Source: three-view drawing plus pictorial views. Frame: mm from the lowest corner of the part. A direction names the side the tool comes from. Give positions to 0.01 mm unless a question says otherwise; leave off trailing zeros. Order: outer loops, then holes, each group sorted by start corner. A loop starts at its lowest first (then second) coordinate and runs counter-clockwise, first axis right, second up. Notation, with made-up numbers: M 36,-18.5 L 83,-18.5 A19 cw 83,-10.5 Z; hole C 16,62.25 d2. An arc over 180 degrees is marked long. Use CSV: the item, a comma, the result in double quotes. Start each with the question number.
1. Section query B-B, the plane x = 24. Return the cut outline in (y, z), plus the area to 3 significant figures.
2. Mould query, pull axis Y, two halves, no side actions, for the marked faces 1, 2, 3 and 4. Classes: released by +Y, released by -Y, zero draft, split by the parting line, or undercut.
3. Section query A-A, the plane z = 12. Return the cut outline in (x, y), plus the area to 3 significant figures.
4. Section query C-C, the plane y = 24. Return the cut outline in (x, z), plus the area to 3 significant figures.
5. Reachability of the marked faces 5, 6 and 7 from +Z, -Z, +X, -X, +Y, -Y: full face, straight path, thin tool, end or side. Return the list, or none.
6. Line query: line 1 along Z through (x, y) = (24, 28.45); line 2 along Y through (x, z) = (23, 9.5); line 3 along Y through (x, z) = (36.5, 38). Output: solid intervals per line, ascending. Write a range as [from, to].
7. Section query D-D, the plane z = 4.5. Return the cut outline in (x, y).
8. Pin query (flat end, axial travel): P1, Ø6, axis at x = 26.5, z = 6.5, coming from the -Y side; P2, Ø1.5, axis at y = 20, z = 13.5, coming from the +X side; P3, Ø10, axis at x = 37, z = 13.5, coming from the -Y side; P4, Ø22, axis at x = 26, y = 23.5, coming from the -Z side. Return the tip coordinate at first contact, or that it passes through.
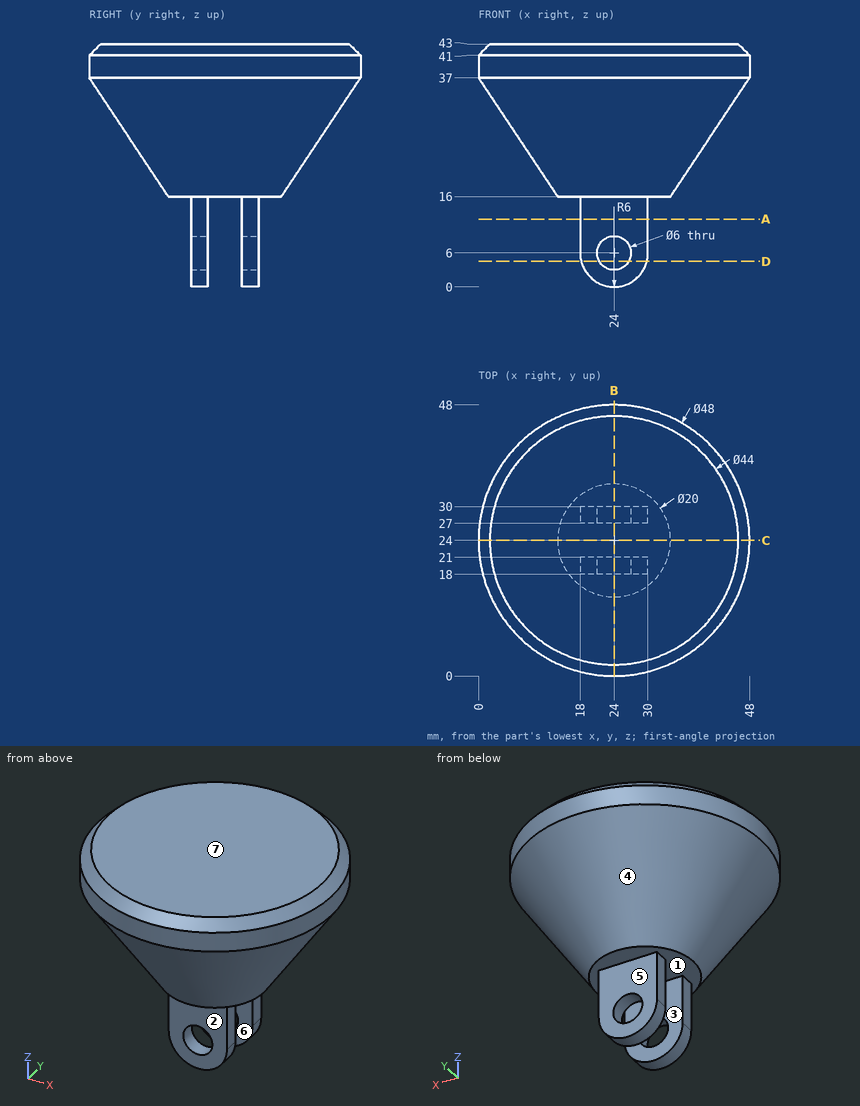
Result set:
1,outline,"M 0,37 L 14,16 L 18,16 L 18,9 L 21,9 L 21,16 L 27,16 L 27,9 L 30,9 L 30,16 L 34,16 L 48,37 L 48,41 L 46,43 L 2,43 L 0,41 Z; M 18,0 L 21,0 L 21,3 L 18,3 Z; M 27,0 L 30,0 L 30,3 L 27,3 Z"
1,area,"1,060 mm2"
2,face 1,"undercut"
2,face 2,"released by -Y"
2,face 3,"undercut"
2,face 4,"split by the parting line"
3,outline,"M 18,18 L 30,18 L 30,21 L 18,21 Z; M 18,27 L 30,27 L 30,30 L 18,30 Z"
3,area,"72.0 mm2"
4,outline,"M 0,37 L 14,16 L 34,16 L 48,37 L 48,41 L 46,43 L 2,43 L 0,41 Z"
4,area,"998 mm2"
5,face 5,"-Z, +X, -X, +Y"
5,face 6,"-Z, +X, -X"
5,face 7,"+Z, +X, -X, +Y, -Y"
6,line 1,"[0, 3], [9, 43]"
6,line 2,"[18, 21], [27, 30]"
6,line 3,"[3.51, 44.49]"
7,outline,"M 18.19,18 L 21.4,18 L 21.4,21 L 18.19,21 Z; M 18.19,27 L 21.4,27 L 21.4,30 L 18.19,30 Z; M 26.6,18 L 29.81,18 L 29.81,21 L 26.6,21 Z; M 26.6,27 L 29.81,27 L 29.81,30 L 26.6,30 Z"
8,P1,"y = 18"
8,P2,"x = 30"
8,P3,"y = 18.92"
8,P4,"z = 0"
